Build history of the part. All positions in model axes, mm. Face numbers are marked on the shaded views. Round coordinates to 2 decimals unless told otherwise and drop trailing zeros. Write each loop counter-clockwise with the first axis right and the second up, starting at its lowest first coordinate (ties: lowest second). Pieces come first, ordered by that corner, then holes. Notation, with made-up numbers: M 20,32.5 L 45,32.5 A22 ccw 45,61.5 Z; hole C -22,34.5 d2. An arc over 180 degrees is marked long. Write item = value, one per line.
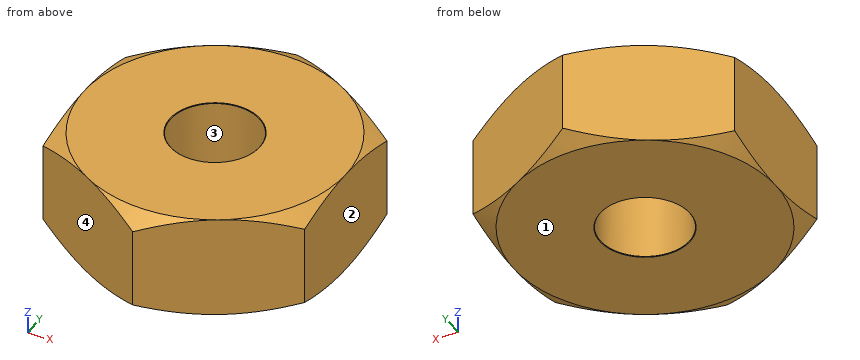
Autodesk Inventor part; units mm, degrees
ref_plane "MSC_PF1" through (0, 0, 0) normal (1, 0, 0) x (0, 1, 0)
ref_plane "MSC_PT1" through (0, 0, 0) normal (0, 0, 1) x (1, 0, 0)
ref_plane "YZ Plane" through (0, 0, 0) normal (1, 0, 0) x (0, 1, 0)
sketch "Sketch7" plane through (0, 0, 0) normal (0, 0, 1) x (1, 0, 0)
  circle A0 centre (0, 0) radius 3.175 construction
  line L0 (-3.175, -1.8331) -> (-3.175, 1.8331)
  line L1 (-3.175, 1.8331) -> (0, 3.6662)
  line L2 (0, 3.6662) -> (3.175, 1.8331)
  line L3 (3.175, 1.8331) -> (3.175, -1.8331)
  line L4 (3.175, -1.8331) -> (0, -3.6662)
  line L5 (0, -3.6662) -> (-3.175, -1.8331)
  dimension "d40" = 6.35
extrude "Extrusion1" add sketch "Sketch7" against normal blind 2.4892
sketch "Sketch11" plane through (0, 0, 0) normal (0, 0, 1) x (1, 0, 0)
  line L0 (0, 3.6662) -> (3.175, 1.8331)
  line L1 (-3.175, 1.8331) -> (0, 3.6662)
  line L2 (-3.175, 1.8331) -> (3.175, -1.8331) construction
  line L3 (-3.175, -1.8331) -> (3.175, 1.8331) construction
  point P0 (0, 0)
hole "Hole1" at (0, 0, 0) direction (0, 0, -1) diameter 2.1565 end through all
chamfer "Chamfer1" distance 0.0125 angle 45 2 edges at (0, 1.0782, 0) (0, 1.0782, -2.4892)
sketch "Sketch9" plane through (0, 0, 0) normal (1, 0, 0) x (0, 1, 0)
  line L0 (-3.6662, -2.2056) -> (-3.6662, -2.4892)
  line L1 (-3.6662, -2.4892) -> (-3.175, -2.4892)
  line L2 (-3.175, -2.4892) -> (-3.6662, -2.2056)
  line L3 (0, -2.5459) -> (0, -2.1489)
  line L4 (-3.6662, -2.4892) -> (-1.8331, -2.4892)
  dimension "d38" = 6.35
  dimension "d41" = 150
revolve "Revolution1" cut sketch "Sketch9" angle 360 about axis through (0, 0, -10) along (0, 0, 1)
sketch "Sketch10" plane through (0, 0, 0) normal (1, 0, 0) x (0, 1, 0)
  line L0 (-3.6662, -0.2836) -> (-3.6662, 0)
  line L1 (-3.6662, 0) -> (-3.175, 0)
  line L2 (-3.175, 0) -> (-3.6662, -0.2836)
  line L3 (0, -0.3403) -> (0, 0.0567)
  line L4 (-1.8331, 0) -> (-3.6662, 0)
  dimension "d45" = 6.35
  dimension "d46" = 150
revolve "Revolution2" cut sketch "Sketch10" angle 360 about axis through (0, 0, -10) along (0, 0, 1)
ref_plane "MSC_PF1" through (0, 0, 0) normal (1, 0, 0) x (0, 1, 0)
ref_plane "MSC_PT1" through (0, 0, 0) normal (0, 0, 1) x (1, 0, 0)
equation "\"d38\" = Fbas"
equation "\"d40\" = Fbas"
equation "\"d29\" = Hbas"
equation "\"d63\" = 0.5 * PTC"
equation "\"d45\" = Fbas"
equation "\"Fbas\" = 6.35"
equation "\"Hbas\" = 2.4892"
equation "\"NND\" = 2.8448"
equation "\"THREADDIA\" = NND"
properties part number "ASME B18.6.3 - 4-40" material "Steel, Mild"
1. Band-saw the part on B-B (z = -0.15). List the corners of the cut face in (x, y) (1 decimal).
Responses:
outline = M -3.2,-1.3 A3.4 ccw -2.7,-2.1 L -0.5,-3.4 A3.4 ccw 0.5,-3.4 L 2.7,-2.1 A3.4 ccw 3.2,-1.3 L 3.2,1.3 A3.4 ccw 2.7,2.1 L 0.5,3.4 A3.4 ccw -0.5,3.4 L -2.7,2.1 A3.4 ccw -3.2,1.3 Z; hole C 0,0 d2.2
2. Flat gauge pin, fed straight in: pin 1 (1.3 mm diameter, centred on x = 0, y = 0, fed in from -Z). Where does the tip first touch, or does it go through?
Responses:
pin_1 = through
3. Probe probe 1 along X at (y, z) = (0, -2.1) (3 decimals); probe 2 along Y at (x, z) = (0.5, -1.45); probe 3 along X at (y, z) = (-0.25, -1.2) (3 decimals). List the from-to ranges inside material, lowest first.
Responses:
probe_1 = -3.175 to -1.078, 1.078 to 3.175
probe_2 = -3.38 to -0.96, 0.96 to 3.38
probe_3 = -3.175 to -1.049, 1.049 to 3.175
4. Mould opens along X. For the marked faces 1, 2, 3 and 4 say: pulls with the +X half, pulls with the -X half, needs draft (parallel to the pull), parting line crosses it, or undercut.
Responses:
face_1 = needs draft
face_2 = pulls with the +X half
face_3 = undercut
face_4 = pulls with the -X half
5. Band-saw the part on A-A (z = -1.9). List the corners of the cut face in (x, y) (1 decimal), plus the area to 3 significant figures.
Responses:
outline = M -3.2,-1.8 L 0,-3.7 L 3.2,-1.8 L 3.2,1.8 L 0,3.7 L -3.2,1.8 Z; hole C 0,0 d2.2
area = 31.3 mm²
